from build123d import *

# Parameters (mm, degrees)
F0_W      = 67.7789226174
F0_H      = 110.2438345551
F1_DEPTH  = 10.668
F2_W      = 67.7789226174
F2_H      = 21.9810828567
F3_DEPTH  = 84.074
F4_DEPTH  = 15.748
F5_DEPTH  = 34.544
F7_DEPTH  = 25.4
F9_DEPTH  = 64.77
F10_W     = 32.31433779
F10_H     = 40.7657716423
F11_DEPTH = 30.48


with BuildPart() as f1:
    # F0 (on Top) → F1 (new body)
    with BuildSketch(Plane.XY):
        Rectangle(F0_W, F0_H)
    extrude(amount=F1_DEPTH)

    # F2 (on face) → F3 (join)
    with BuildSketch(Plane.XY.offset(10.668)):
        with Locations((0, 44.1313758492)):
            Rectangle(F2_W, F2_H)
    extrude(amount=F3_DEPTH)

    # F4 (add): a face of the model
    f4_faces = [f1.faces().sort_by_distance(p)[0] for p in [
        (0, -10.9905414283, 10.668),
    ]]
    extrude(f4_faces, amount=F4_DEPTH)

    # F5 (add): a face of the model
    f5_faces = [f1.faces().sort_by_distance(p)[0] for p in [
        (0, 44.1313758492, 94.742),
    ]]
    extrude(f5_faces, amount=F5_DEPTH)

    # F6 (on face) → F7 (cut)
    with BuildSketch(Plane.XZ.offset(-33.1408344209)):
        with BuildLine():
            Line((6.9014118053, 129.286), (-9.5512475818, 129.286))
            Line((-9.5512475818, 129.286), (-9.5512475818, 92.9261893034))
            ThreePointArc((-9.5512475818, 92.9261893034), (-1.3249178883, 84.6998596098), (6.9014118053, 92.9261893034))
            Line((6.9014118053, 92.9261893034), (6.9014118053, 129.286))
        make_face()
    extrude(amount=-F7_DEPTH, mode=Mode.SUBTRACT)

    # F8 (on face) → F9 (cut)
    with BuildSketch(Plane.XY.offset(26.416)):
        with BuildLine():
            ThreePointArc((33.8894613087, -22.0553063396), (0.997184828, -54.9834271284), (-33.8894613087, -24.1762053761))
            Line((-33.8894613087, -24.1762053761), (-33.8894613087, -55.1219172776))
            Line((-33.8894613087, -55.1219172776), (33.8894613087, -55.1219172776))
            Line((33.8894613087, -55.1219172776), (33.8894613087, -22.0553063396))
        make_face()
    extrude(amount=-F9_DEPTH, mode=Mode.SUBTRACT)

    # F10 (on face) → F11 (cut)
    with BuildSketch(Plane.YZ.offset(33.8894613087)):
        with Locations((43.3757714927, 15.2329867706)):
            Rectangle(F10_W, F10_H)
    extrude(amount=-F11_DEPTH, mode=Mode.SUBTRACT)


solid = f1.part
Geometry check sheet. Reference: the model listing, model coordinates, mm. A direction names the side the tool comes from. Coordinates: 2 decimals unless noted, no trailing zeros. Order: outer loops, then holes, each group sorted by start corner. A loop starts at its lowest first (then second) coordinate and runs counter-clockwise, first axis right, second up. Notation, with made-up numbers: M 65.25,-25.5 L 90.25,-25.5 A23 cw 90.25,-17.5 Z; hole C -21,15.25 d1. An arc over 180 degrees is marked long. Use CSV: the item, a comma, the result in double quotes.
Item 1: Thickness scan on line 1 along X through (y, z) = (48, 33.5); line 2 along Z through (x, y) = (-5, -17); line 3 along Y through (x, z) = (15, 118). Record the ranges inside material, lowest first.
Returned:
line 1,"x = -33.89 to 3.41"
line 2,"z = 0 to 26.42"
line 3,"y = 33.14 to 55.12"
Item 2: Tool access check on faces 1 (the flat face through (6.901, 44, 111)), 2 (the flat face through (19, 27.219, 13)), 3 (the flat face through (0, -10, 26.416)), 4 (the flat face through (3.409, 41, 18)). Record the directions out of +Z, -Z, +X, -X, +Y, -Y that give a thin tool (end or side, any length) a straight path to the whole face; none if there is none.
Returned:
face 1,"+Z, +Y, -Y"
face 2,"+Z, -Z, +X, +Y"
face 3,"+Z, +X, -X, -Y"
face 4,"-Z, +X, +Y"
Item 3: Cross-section at C-C on x = -28. Record the cut outline in (y, z), then the cut area to 3 significant figures.
Returned:
outline,"M -40.36,0 L 55.12,0 L 55.12,129.29 L 33.14,129.29 L 33.14,26.42 L -40.36,26.42 Z"
area,"4,780 mm2"
Item 4: Cross-section at A-A on x = 30. Record the cut outline in (y, z), then the cut area to 3 significant figures.
Returned:
outline,"M -36.84,0 L 27.22,0 L 27.22,26.42 L -36.84,26.42 Z; M 33.14,35.62 L 55.12,35.62 L 55.12,129.29 L 33.14,129.29 Z"
area,"3,750 mm2"
Item 5: Cross-section at B-B on z = 9. Record the cut outline in (x, y), then the cut area to 3 significant figures.
Returned:
outline,"M -33.89,-24.18 A33.97 ccw 33.89,-22.06 L 33.89,27.22 L 3.41,27.22 L 3.41,55.12 L -33.89,55.12 Z"
area,"6,120 mm2"
Item 6: Cross-section at D-D on y = 7. Record the cut outline in (x, z), then the cut area to 3 significant figures.
Returned:
outline,"M -33.89,0 L 33.89,0 L 33.89,26.42 L -33.89,26.42 Z"
area,"1,790 mm2"
Item 7: Gauge pin test, flat ends, axial feed: pin 1 Ø14 at (y, z) = (46.5, 26.5) entering from +X; pin 2 Ø2 at (x, y) = (17.5, -3.5) entering from +Z; pin 3 Ø8 at (x, z) = (21, 16.5) entering from +Y. Record the tip position at first contact, or that the pin passes through.
Returned:
pin 1,"stops at x = 3.41"
pin 2,"stops at z = 26.42"
pin 3,"stops at y = 27.22"
